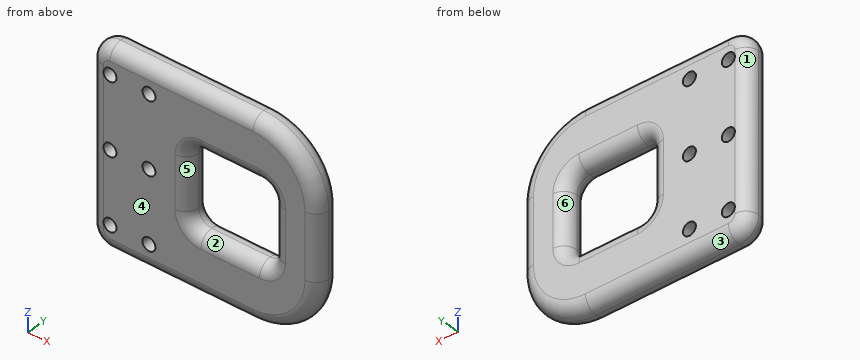
from build123d import *

# Parameters (mm, degrees)
SKETCH1_R           = 1
BOSS_EXTRUDE1_DEPTH = 2
FILLET1_R           = 2


with BuildPart() as part:
    # Sketch1 → Boss-Extrude1 (new, symmetric)
    with BuildSketch(Plane(origin=(0, 0, 0), x_dir=(1, 0, 0), z_dir=(0, 1, 0))):
        with BuildLine():
            Line((-14.5, 15), (7.5, 15))
            ThreePointArc((7.5, 15), (14.571067812, 12.071067812), (17.5, 5))
            Line((17.5, 5), (17.5, -5))
            ThreePointArc((17.5, -5), (14.571067812, -12.071067812), (7.5, -15))
            Line((7.5, -15), (-14.5, -15))
            ThreePointArc((-14.5, -15), (-16.621320344, -14.121320344), (-17.5, -12))
            Line((-17.5, -12), (-17.5, 12))
            ThreePointArc((-17.5, 12), (-16.621320344, 14.121320344), (-14.5, 15))
        make_face()
        with Locations(Location((-8.5, 11, 0), (0, 0, 270))):
            Circle(SKETCH1_R, mode=Mode.SUBTRACT)
        with Locations(Location((-14.5, 11, 0), (0, 0, 270))):
            Circle(SKETCH1_R, mode=Mode.SUBTRACT)
        with Locations(Location((-14.5, -11, 0), (0, 0, 270))):
            Circle(SKETCH1_R, mode=Mode.SUBTRACT)
        with Locations(Location((-8.5, -11, 0), (0, 0, 270))):
            Circle(SKETCH1_R, mode=Mode.SUBTRACT)
        with Locations(Location((-8.5, 0, 0), (0, 0, 270))):
            Circle(SKETCH1_R, mode=Mode.SUBTRACT)
        with Locations(Location((-14.5, 0, 0), (0, 0, 270))):
            Circle(SKETCH1_R, mode=Mode.SUBTRACT)
        with BuildLine():
            Line((-0.5, 6), (8.5, 6))
            ThreePointArc((8.5, 6), (9.914213562, 5.414213562), (10.5, 4))
            Line((10.5, 4), (10.5, -4))
            ThreePointArc((10.5, -4), (9.914213562, -5.414213562), (8.5, -6))
            Line((8.5, -6), (-0.5, -6))
            ThreePointArc((-0.5, -6), (-1.914213562, -5.414213562), (-2.5, -4))
            Line((-2.5, -4), (-2.5, 4))
            ThreePointArc((-2.5, 4), (-1.914213562, 5.414213562), (-0.5, 6))
        make_face(mode=Mode.SUBTRACT)
    extrude(amount=BOSS_EXTRUDE1_DEPTH, both=True)

    # Fillet1
    fillet1_edges = [part.edges().sort_by_distance(p)[0] for p in [
        (14.571067812, -2, 12.071067812),
        (-3.5, -2, 15),
        (-16.621320344, -2, 14.121320344),
        (-17.5, -2, 0),
        (-16.621320344, -2, -14.121320344),
        (-3.5, -2, -15),
        (14.571067812, -2, -12.071067812),
        (14.571067812, 2, 12.071067812),
        (-3.5, 2, 15),
        (-16.621320344, 2, 14.121320344),
        (-17.5, 2, 0),
        (-16.621320344, 2, -14.121320344),
        (-3.5, 2, -15),
        (14.571067812, 2, -12.071067812),
        (9.914213562, -2, 5.414213562),
        (4, -2, 6),
        (-1.914213562, -2, 5.414213562),
        (-2.5, -2, 0),
        (-1.914213562, -2, -5.414213562),
        (4, -2, -6),
        (9.914213562, -2, -5.414213562),
        (-1.914213562, 2, -5.414213562),
        (4, 2, -6),
        (9.914213562, 2, -5.414213562),
        (10.5, 2, 0),
        (9.914213562, 2, 5.414213562),
        (4, 2, 6),
        (-1.914213562, 2, 5.414213562),
        (17.5, -2, 0),
        (17.5, 2, 0),
        (10.5, -2, 0),
        (-2.5, 2, 0),
    ]]
    fillet(fillet1_edges, radius=FILLET1_R - 0.0001)  # a hair under: the kernel refuses the full size


solid = part.part
Can you work these out from the model? Positions are in its coordinate system, mm. Face numbers are marked on the shaded views. A direction names the side the tool comes from. Give positions to 0.01 mm unless a question says otherwise; leave off trailing zeros. Return JSON: item names as keys, results as strings.
1. We'd pull the mould along Z, two halves only. Please class the marked faces 1, 2 and 3: +Z half, -Z half, draft (parallel to the pull), parting line (faces both ways), or undercut.
Output values:
{"face 1": "draft", "face 2": "undercut", "face 3": "-Z half"}
2. For the marked faces 4, 5 and 6, which set-ups out of +Z, -Z, +X, -X, +Y, -Y let a thin tool reach every point of the face, with its end or its side?
Output values:
{"face 4": "+Z, -Z, +X, -X, -Y", "face 5": "-Y", "face 6": "+Y"}
3. If I drill on line 1 (X direction, y = -0.1, z = 11); line 2 (X direction, y = 0.85, z = -11); line 3 (Z direction, x = 7, y = -0.2), over which ranges is the centre line in solid material (lowest first)?
Output values:
{"line 1": "x = -17.5 to -15.5, -13.5 to -9.5, -7.5 to 15.5", "line 2": "x = -17.31 to -15.5, -13.5 to -9.5, -7.5 to 15.26", "line 3": "z = -14.99 to -6.01, 6.01 to 14.99"}
4. I want a section at B-B on z = 0. Give the number of separate pieces and of enclosed holes in the cut face, and give its area (3 significant figures).
Output values:
{"separate pieces": "4", "enclosed holes": "0", "area": "65.1 mm²"}
5. I'm going to push flat-ended pins straight in: pin 1 Ø1.5 at (x, z) = (-1.5, 6.5) entering from -Y; pin 2 Ø1.5 at (x, y) = (13, -1) entering from +Z; pin 3 Ø2 at (x, y) = (11, 1.5) entering from -Z. Where does each tip first touch, or does it pass through?
Output values:
{"pin 1": "stops at y = -1.92", "pin 2": "stops at z = 13.63", "pin 3": "stops at z = -14.44"}
